Geometry check sheet. Reference: the model listing, model coordinates, mm. Face numbers are marked on the shaded views. A direction names the side the tool comes from. Round coordinates to 2 decimals unless told otherwise and drop trailing zeros. Order: outer loops, then holes, each group sorted by start corner. A loop starts at its lowest first (then second) coordinate and runs counter-clockwise, first axis right, second up.
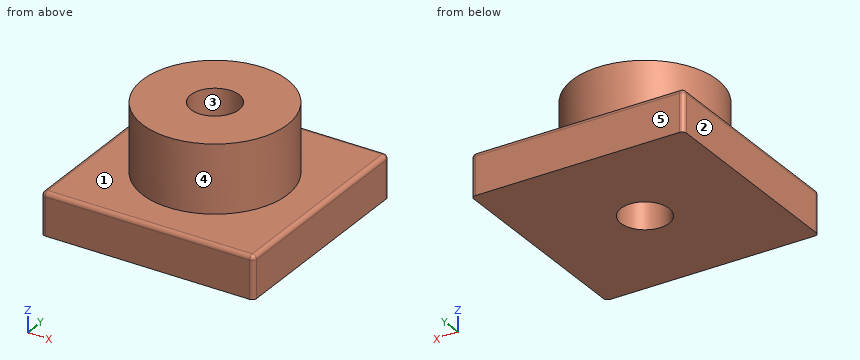
```python
from build123d import *

# Parameters (mm, degrees)
F0_W     = 256.570498
F0_H     = 256.570498
F0_R     = 29.163007
F1_DEPTH = 50.8
F2_R     = 5.08
F3_R     = 5.08
F4_R     = 5.08
F5_R     = 5.08
F6_R     = 87.489022
F6_R_2   = 29.163007
F7_DEPTH = 132.588


with BuildPart() as f1:
    # F0 (on Top) → F1 (new body)
    with BuildSketch(Plane.XY):
        Rectangle(F0_W, F0_H)
        Circle(F0_R, mode=Mode.SUBTRACT)
    extrude(amount=F1_DEPTH)

    # F2
    f2_edges = [f1.edges().sort_by_distance(p)[0] for p in [
        (0, 128.285249, 50.8),
    ]]
    fillet(f2_edges, radius=F2_R)

    # F3
    f3_edges = [f1.edges().sort_by_distance(p)[0] for p in [
        (128.285249, -2.54, 50.8),
    ]]
    fillet(f3_edges, radius=F3_R)

    # F4
    f4_edges = [f1.edges().sort_by_distance(p)[0] for p in [
        (-2.54, -128.285249, 50.8),
    ]]
    fillet(f4_edges, radius=F4_R)

    # F5
    f5_edges = [f1.edges().sort_by_distance(p)[0] for p in [
        (-128.285249, 0, 50.8),
    ]]
    fillet(f5_edges, radius=F5_R)

    # F6 (on Top) → F7 (join)
    with BuildSketch(Plane.XY):
        Circle(F6_R)
        Circle(F6_R_2, mode=Mode.SUBTRACT)
    extrude(amount=F7_DEPTH)


solid = f1.part
```
(1) Draft check along X on the marked faces 3, 4 and 5. Enter one of: released by +X, released by -X, zero draft, split by the parting line, or undercut.
Returned:
face 3: undercut
face 4: split by the parting line
face 5: zero draft
(2) Depth check by flat-ended pin: P1, Ø6, axis at y = 60, z = 115, coming from the -X side; P2, Ø2, axis at x = 11, z = 62.5, coming from the +Y side; P3, Ø6, axis at x = -55, z = 107.5, coming from the +Y side. Enter the tip coordinate at first touch or a pass-through.
Returned:
P1: stops at x = -66.37
P2: stops at y = 86.92
P3: stops at y = 70.36
(3) Material ranges on line 1 (Y direction, x = 0, z = 73.5); line 2 (Y direction, x = 0, z = 33); line 3 (Z direction, x = -114, y = 88), recorded low to high.
Returned:
line 1: y = -87.49 to -29.16, 29.16 to 87.49
line 2: y = -128.29 to -29.16, 29.16 to 128.29
line 3: z = 0 to 50.8
(4) Sectioned sample at C-C, the plane x = 103. Record the cut outline in (y, z), and give its area (3 significant figures).
Returned:
outline: (-128.29, 0) - (128.29, 0) - (128.29, 45.72) arc R5.08 ccw to (123.21, 50.8) - (-123.21, 50.8) arc R5.08 ccw to (-128.29, 45.72) - close
area: 13,000 mm2
(5) Set-up check for the marked faces 1 and 2: record each of +Z, -Z, +X, -X, +Y, -Y from which the full face is reachable in a straight line by a thin tool's end or side.
Returned:
face 1: +Z
face 2: +Z, -Z, -X, +Y, -Y
(6) Sectioned sample at A-A, the plane x = 0. Record the cut outline in (y, z), and give its area (3 significant figures).
Returned:
outline: (-128.29, 0) - (-29.16, 0) - (-29.16, 132.59) - (-87.49, 132.59) - (-87.49, 50.8) - (-123.21, 50.8) arc R5.08 ccw to (-128.29, 45.72) - close; (29.16, 0) - (128.29, 0) - (128.29, 45.72) arc R5.08 ccw to (123.21, 50.8) - (87.49, 50.8) - (87.49, 132.59) - (29.16, 132.59) - close
area: 19,600 mm2
(7) Sectioned sample at B-B, the plane y = 19.5. Record the cut outline in (x, z), and give its area (3 significant figures).
Returned:
outline: (-128.29, 0) - (-21.68, 0) - (-21.68, 132.59) - (-85.29, 132.59) - (-85.29, 50.8) - (-123.21, 50.8) arc R5.08 ccw to (-128.29, 45.72) - close; (21.68, 0) - (128.29, 0) - (128.29, 45.72) arc R5.08 ccw to (123.21, 50.8) - (85.29, 50.8) - (85.29, 132.59) - (21.68, 132.59) - close
area: 21,200 mm2
